```python
from build123d import *

# Parameters (mm, degrees)
Y_KSEKLIK_EKSTR_ZYON1_START = -315
IZIM2_R                     = 15
Y_KSEKLIK_EKSTR_ZYON1_DEPTH = 3
Y_KSEKLIK_EKSTR_ZYON2_START = 312
IZIM2_2_R                   = 15
Y_KSEKLIK_EKSTR_ZYON2_DEPTH = 3
KES_EKSTR_ZYON2_DEPTH       = 15
KES_EKSTR_ZYON3_START       = -600
KES_EKSTR_ZYON3_DEPTH       = 30


with BuildPart() as part:
    # izim1 → D_nd_r1 (revolve)
    with BuildSketch(Plane.XY, mode=Mode.PRIVATE) as d_nd_r1_sk:
        Polygon((450, 0), (450, 7), (432.5, 7), (432.5, 10), (395, 10), (395, 12.5), (-395, 12.5), (-395, 10), (-432.5, 10), (-432.5, 7), (-450, 7), (-450, 0), align=None)
    revolve(d_nd_r1_sk.sketch.rotate(Axis((-450, 0, 0), (1, 0, 0)), 90), axis=Axis((-450, 0, 0), (1, 0, 0)))

    # izim2 → Y_kseklik-Ekstr_zyon1 (add)
    with BuildSketch(Plane(origin=(0, 0, 0), x_dir=(0, 0, -1), z_dir=(1, 0, 0)).offset(Y_KSEKLIK_EKSTR_ZYON1_START)):
        Circle(IZIM2_R)
    extrude(amount=Y_KSEKLIK_EKSTR_ZYON1_DEPTH)

    # izim2_2 → Y_kseklik-Ekstr_zyon2 (add)
    with BuildSketch(Plane(origin=(0, 0, 0), x_dir=(0, 0, -1), z_dir=(1, 0, 0)).offset(Y_KSEKLIK_EKSTR_ZYON2_START)):
        Circle(IZIM2_2_R)
    extrude(amount=Y_KSEKLIK_EKSTR_ZYON2_DEPTH)

    # izim4 → Kes-Ekstr_zyon2 (cut, symmetric)
    with BuildSketch(Plane(origin=(0, 0, 0), x_dir=(0, 0, -1), z_dir=(1, 0, 0))):
        with BuildLine():
            Line((-12.459935794, 1), (-1, 1))
            Line((-1, 1), (-1, 12.459935794))
            ThreePointArc((-1, 12.459935794), (0, 12.5), (1, 12.459935794))
            Line((1, 12.459935794), (1, 1))
            Line((1, 1), (12.459935794, 1))
            ThreePointArc((12.459935794, 1), (12.5, 0), (12.459935794, -1))
            Line((12.459935794, -1), (1, -1))
            Line((1, -1), (1, -12.459935794))
            ThreePointArc((1, -12.459935794), (0, -12.5), (-1, -12.459935794))
            Line((-1, -12.459935794), (-1, -1))
            Line((-1, -1), (-12.459935794, -1))
            ThreePointArc((-12.459935794, -1), (-12.5, 0), (-12.459935794, 1))
        make_face()
    extrude(amount=KES_EKSTR_ZYON2_DEPTH, both=True, mode=Mode.SUBTRACT)

    # izim6 → Kes-Ekstr_zyon3 (cut)
    with BuildSketch(Plane(origin=(450, 0, 0), x_dir=(0, 0, -1), z_dir=(1, 0, 0)).offset(KES_EKSTR_ZYON3_START)):
        with BuildLine():
            Line((1, 1), (1, 12.459935794))
            ThreePointArc((1, 12.459935794), (0, 12.5), (-1, 12.459935794))
            Line((-1, 12.459935794), (-1, 1))
            Line((-1, 1), (-12.459935794, 1))
            ThreePointArc((-12.459935794, 1), (-12.5, 0), (-12.459935794, -1))
            Line((-12.459935794, -1), (-1, -1))
            Line((-1, -1), (-1, -12.459935794))
            ThreePointArc((-1, -12.459935794), (0, -12.5), (1, -12.459935794))
            Line((1, -12.459935794), (1, -1))
            Line((1, -1), (12.459935794, -1))
            ThreePointArc((12.459935794, -1), (12.5, 0), (12.459935794, 1))
            Line((12.459935794, 1), (1, 1))
        make_face()
    extrude(amount=KES_EKSTR_ZYON3_DEPTH, mode=Mode.SUBTRACT)


solid = part.part
```
Here's how the part is built. I have some questions about the finished solid (model axes, mm). A direction names the side the tool comes from. Coordinates: 2 decimals unless noted, no trailing zeros. Order: outer loops, then holes, each group sorted by start corner. A loop starts at its lowest first (then second) coordinate and runs counter-clockwise, first axis right, second up. Notation, with made-up numbers: (81, -2) -> (128, -2) arc R29 cw to (128, 19) -> close; hole circle Ø6 at (32, -12). An arc over 180 degrees is marked (long way). Return JSON: item names as keys, results as strings.
1) I'm going to push flat-ended pins straight in: P1, Ø9, axis at x = -3.5, y = -6.5, coming from the -Z side; P2, Ø4, axis at y = -0.5, z = -11.5, coming from the +X side; P3, Ø3.5, axis at x = -129.5, z = -7.5, coming from the +Y side; P4, Ø12, axis at y = 1.5, z = -10.5, coming from the -X side. Where does each tip first touch, or does it pass through?
Conclusion:
{"P1": "stops at z = -12.34", "P2": "stops at x = 432.5", "P3": "stops at y = 11.1", "P4": "stops at x = -450"}
2) If we section it at A-A on x = 205: List the corners of the cut face in (y, z) for me, plus the area to 3 significant figures.
Conclusion:
{"outline": "circle Ø25 at (0, 0)", "area": "491 mm²"}
3) If I drill on probe 1 along X at (y, z) = (0, 3.5); probe 2 along X at (y, z) = (3.25, -12.75); probe 3 along X at (y, z) = (-5.25, 7.75), over which ranges is the centre line in solid material (lowest first)?
Conclusion:
{"probe 1": "x = -450 to -150, -120 to -15, 15 to 450", "probe 2": "x = -315 to -312, 312 to 315", "probe 3": "x = -432.5 to 432.5"}
4) Thinking about a two-plate mould opening in Z: for faces 6 (the cylindrical face through (-441.37, 6.21, 3.23)), 7 (the flat face through (-315, 12.3, 3.4)), 8 (the flat face through (-120, 0, 0)), which applies, +Z half, -Z half, draft (parallel to the pull), parting line (faces both ways), or undercut?
Conclusion:
{"face 6": "parting line", "face 7": "draft", "face 8": "undercut"}
5) On a 3-axis mill with a long thin cutter (end or side, diameter ignored), from which of +Z, -Z, +X, -X, +Y, -Y can I reach the whole of each face in a straight line? I mean faces 1 (the flat face through (-450, 0, 0)), 2 (the cylindrical face through (313.479, 0.66, 14.985)), 3 (the flat face through (-150, 0, 0)), 4 (the flat face through (432.5, -7, -2)), 5 (the flat face through (-395, -10.2, -0.1)). Say none if no direction works.
Conclusion:
{"face 1": "+Z, -Z, -X, +Y, -Y", "face 2": "+X, -X", "face 3": "none", "face 4": "+X", "face 5": "-X"}
